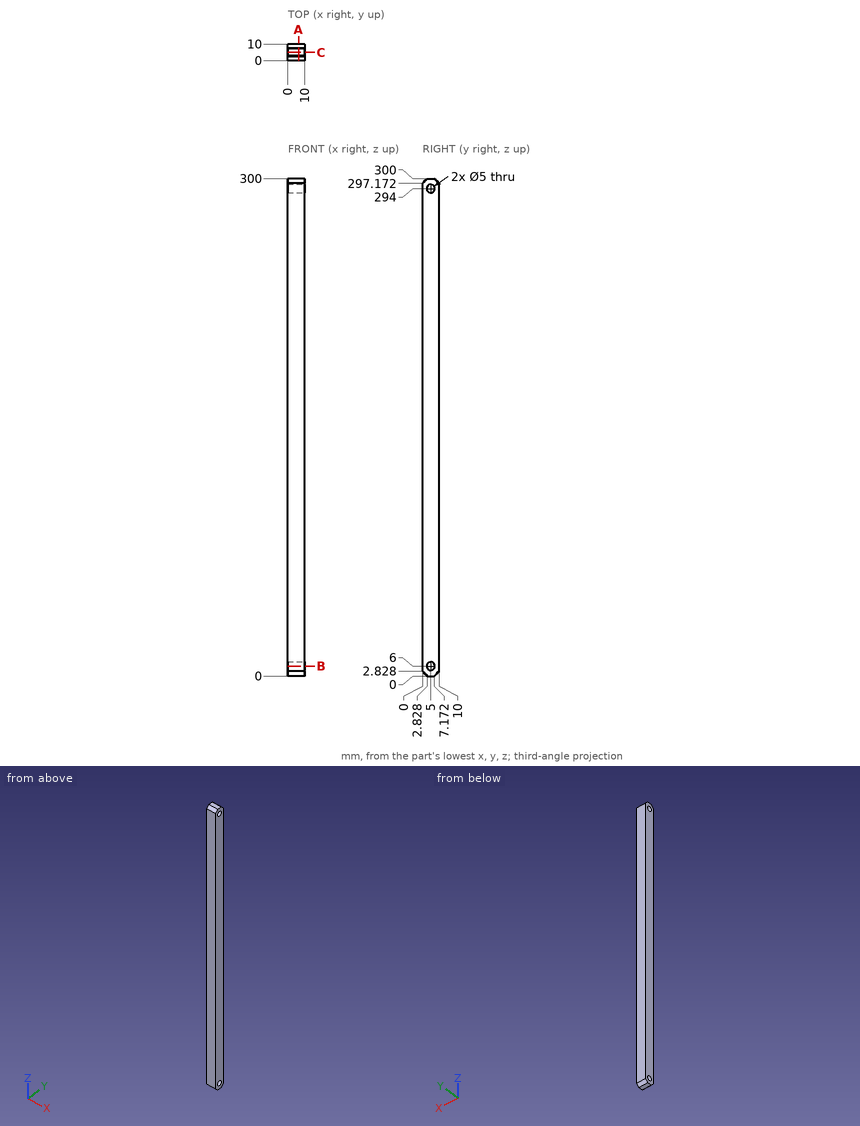
Design review of the part shown in the three views and the two pictorial views. Dimensions are in mm from the part's minimum x, y and z. Coordinates: 2 decimals unless noted, no trailing zeros. Write each loop counter-clockwise with the first axis right and the second up, starting at its lowest first coordinate (ties: lowest second). Pieces come first, ordered by that corner, then holes.
1) We need section C-C on y = 5. State the section outline as (x, z) points, then the cut area to 3 significant figures.
2) We need section A-A on x = 6.5. State the section outline as (y, z) points.
3) To check wall thickness, follow probe 1 along Z at (x, y) = (5.5, 5); probe 2 along Y at (x, z) = (7.75, 294); probe 3 along Z at (x, y) = (4.75, 3.25) (1 decimal). State the ranges of each line that lie inside material, in increasing order.
4) We need section B-B on z = 6. State the section outline as (x, y) points, then the cut area to 3 significant figures.
Answer list:
1. outline: (0, 0) - (10, 0) - (10, 3.5) - (0, 3.5) - close; (0, 8.5) - (10, 8.5) - (10, 291.5) - (0, 291.5) - close; (0, 296.5) - (10, 296.5) - (10, 300) - (0, 300) - close
1. area: 2,900 mm2
2. outline: (0, 2.83) - (2.83, 0) - (7.17, 0) - (10, 2.83) - (10, 297.17) - (7.17, 300) - (2.83, 300) - (0, 297.17) - close; hole circle Ø5 at (5, 6); hole circle Ø5 at (5, 294)
3. probe 1: z = 0 to 3.5, 8.5 to 291.5, 296.5 to 300
3. probe 2: y = 0 to 2.5, 7.5 to 10
3. probe 3: z = 0 to 4.2, 7.8 to 292.2, 295.8 to 300
4. outline: (0, 0) - (10, 0) - (10, 2.5) - (0, 2.5) - close; (0, 7.5) - (10, 7.5) - (10, 10) - (0, 10) - close
4. area: 50.0 mm2
